Job drawing, mm, ordinate dimensions from the low corner. One solid piece. A direction names the side the tool comes from. Coordinates: 2 decimals unless noted, no trailing zeros. Loops run counter-clockwise (first coordinate to the right, second up) from the corner with the lowest first, then second, coordinate; pieces in that order, holes last. Notation, with made-up numbers: (-1, 43) - (9, 43) arc R30 ccw to (9, 80) - close; hole circle Ø3 at (-9, 58.5). An arc over 180 degrees is marked (long way). Use a Markdown table: item, result. Add a question column.
1) Band-saw the part on A-A (x = 9). Give the cut face in (y, z), plus the area to 3 significant figures.
2) Pull direction X, two halves, no side cores. Call the marked faces 3, 4 and 5: +X half, -X half, draft (parallel to the pull), parting line (faces both ways), or undercut.
3) Probe probe 1 along X at (y, z) = (9, 6); probe 2 along Y at (x, z) = (11, 11); probe 3 along X at (y, z) = (25.5, 4.75). List the from-to ranges inside material, lowest first. Write a range as [from, to].
4) Drop flat-ended pins along their axis: P1, Ø3, axis at x = 10.5, z = 7, coming from the -Y side; P2, Ø1.5, axis at x = 6, y = 35, coming from the +Z side; P3, Ø1.6, axis at x = 8.5, z = 8.5, coming from the +Y side. Give the stop position or say it passes through.
5) Band-saw the part on D-D (y = 24). Give the cut face in (x, z).
6) Tool access for the marked faces 1 and 2: list every direction of +Z, -Z, +X, -X, +Y, -Y with a clear straight run to the whole face (end or side of a thin tool).
7) Band-saw the part on B-B (z = 13.25). Give the cut face in (x, y).
8) Band-saw the part on C-C (z = 9). Give the cut face in (x, y), plus the area to 3 significant figures.
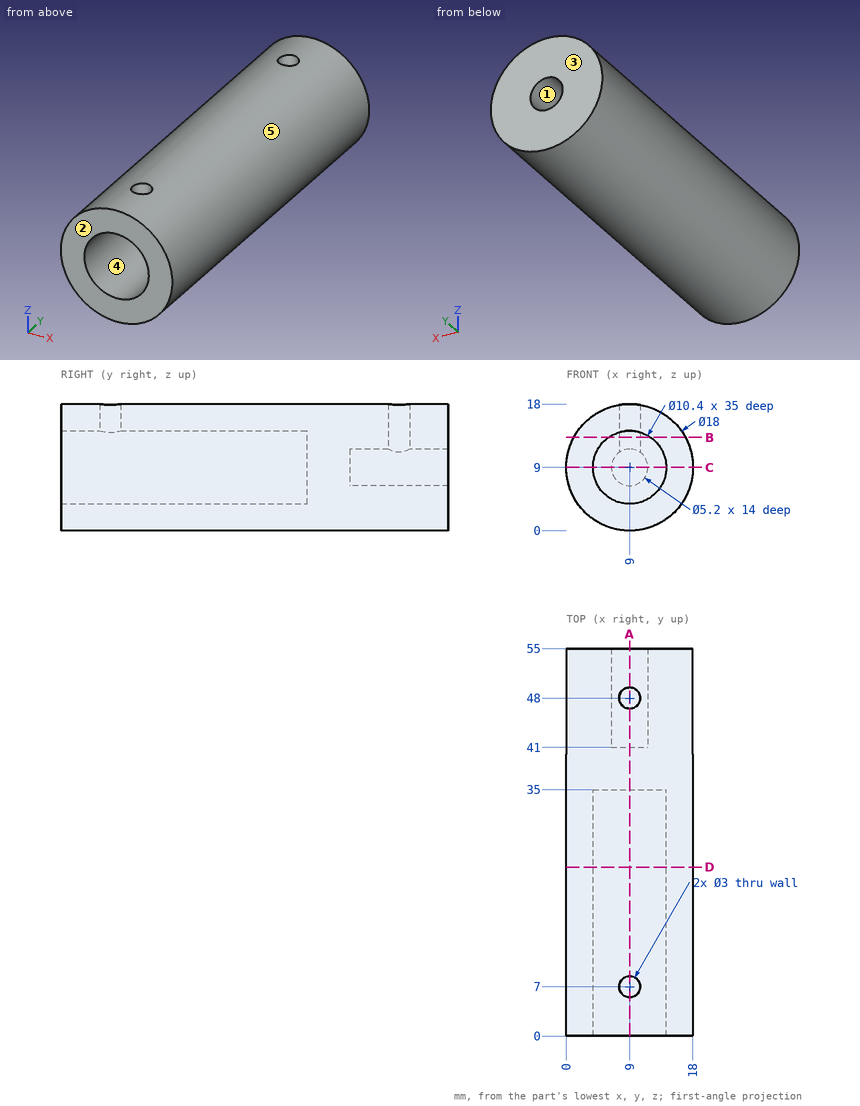
Answer block:
| question | item | result |
|---|---|---|
| 1 | outline | (0, 0) - (55, 0) - (55, 6.4) - (41, 6.4) - (41, 11.6) - (46.5, 11.6) - (46.5, 18) - (8.5, 18) - (8.5, 14.2) - (35, 14.2) - (35, 3.8) - (0, 3.8) - close; (0, 14.2) - (5.5, 14.2) - (5.5, 18) - (0, 18) - close; (49.5, 11.6) - (55, 11.6) - (55, 18) - (49.5, 18) - close |
| 1 | area | 523 mm2 |
| 2 | face 3 | draft |
| 2 | face 4 | undercut |
| 2 | face 5 | parting line |
| 3 | probe 1 | [0.51, 4.75], [13.25, 17.49] |
| 3 | probe 2 | [35, 55] |
| 3 | probe 3 | [1.07, 6], [12, 16.93] |
| 4 | P1 | y = 35 |
| 4 | P2 | z = 17.71 |
| 4 | P3 | y = 41 |
| 5 | outline | circle Ø18 at (9, 9); hole circle Ø10.4 at (9, 9) |
| 6 | face 1 | +Y |
| 6 | face 2 | +Z, -Z, +X, -X, -Y |
| 7 | outline | (1.07, 0) - (6, 0) - (6, 35) - (12, 35) - (12, 0) - (16.93, 0) - (16.93, 55) - (1.07, 55) - close; hole circle Ø3 at (9, 48) |
| 8 | outline | (0, 0) - (3.8, 0) - (3.8, 35) - (14.2, 35) - (14.2, 0) - (18, 0) - (18, 55) - (11.6, 55) - (11.6, 41) - (6.4, 41) - (6.4, 55) - (0, 55) - close |
| 8 | area | 553 mm2 |
